Part model, mm, in its own coordinate system. Give positions to 0.01 mm unless a question says otherwise; leave off trailing zeros. Order: outer loops, then holes, each group sorted by start corner. A loop starts at its lowest first (then second) coordinate and runs counter-clockwise, first axis right, second up.
from build123d import *

# Parameters (mm, degrees)
F0_R        = 4.0800200383
F0_R_2      = 11.0109
F1_DEPTH    = 6.985
F2_T1_DEPTH = 63.627
F2_T4_ANGLE = 170.5132200492
F2_T6_ANGLE = 170.5132200492
F3_T1_DEPTH = 63.627
F3_T4_ANGLE = 170.5132200492
F3_T6_ANGLE = 170.5132200492


# Not quite as in the source:
# - a fillet or chamfer that OpenCascade refuses, or shapes differently, is made with other operations: its cross-section is extruded or revolved along the edge and cut away or added


with BuildPart() as f1:
    # F0 (on Top) → F1 (new body)
    with BuildSketch(Plane.XY):
        with BuildLine():
            Line((28.575, 15.2560200383), (-28.575, 15.2560200383))
            ThreePointArc((-28.575, 15.2560200383), (-40.9829, 0), (-28.575, -15.2560200383))
            Line((-28.575, -15.2560200383), (28.575, -15.2560200383))
            ThreePointArc((28.575, -15.2560200383), (40.9829, 0), (28.575, 15.2560200383))
        make_face()
        with Locations((-12.7, -10.16)):
            Circle(F0_R, mode=Mode.SUBTRACT)
        with Locations((12.7, -10.16)):
            Circle(F0_R, mode=Mode.SUBTRACT)
        with Locations((-25.4, 0)):
            Circle(F0_R_2, mode=Mode.SUBTRACT)
        with Locations((-12.7, 10.16)):
            Circle(F0_R, mode=Mode.SUBTRACT)
        with BuildLine():
            ThreePointArc((-11.0109, 0), (0, 11.0109), (11.0109, 0))
            ThreePointArc((11.0109, 0), (0, -11.0109), (-11.0109, 0))
        make_face(mode=Mode.SUBTRACT)
        with BuildLine():
            ThreePointArc((36.4109, 0), (25.4, -11.0109), (14.3891, 0))
            ThreePointArc((14.3891, 0), (25.4, 11.0109), (36.4109, 0))
        make_face(mode=Mode.SUBTRACT)
        with Locations((12.7, 10.16)):
            Circle(F0_R, mode=Mode.SUBTRACT)
    extrude(amount=F1_DEPTH)

    # F2: fillet of radius 0.762 on 4 edges, made by hand

    # F2_s2 → F2_t1 (cut)
    with BuildSketch(Plane.YZ.offset(-31.8135)):
        with BuildLine():
            ThreePointArc((-14.4940200383, 6.985), (-15.0328354056, 6.7618153673), (-15.2560200383, 6.223))
            Line((-15.2560200383, 6.223), (-15.2560200383, 6.985))
            Line((-15.2560200383, 6.985), (-14.4940200383, 6.985))
        make_face()
        with BuildLine():
            ThreePointArc((15.2560200383, 6.223), (15.0328354056, 6.7618153673), (14.4940200383, 6.985))
            Line((14.4940200383, 6.985), (15.2560200383, 6.985))
            Line((15.2560200383, 6.985), (15.2560200383, 6.223))
        make_face()
    extrude(amount=F2_T1_DEPTH, mode=Mode.SUBTRACT)

    # F2_s3 → F2_t4 (revolve, cut)
    with BuildSketch(Plane(origin=(-25.2263104474, -2.0932144122, 0), x_dir=(0, 0, 1), z_dir=(0.9965750492, 0.0826932365, 0))):
        with BuildLine():
            ThreePointArc((6.985, -16.921308207), (6.7618153673, -17.4601235742), (6.223, -17.683308207))
            Line((6.223, -17.683308207), (6.985, -17.683308207))
            Line((6.985, -17.683308207), (6.985, -16.921308207))
        make_face()
    revolve(axis=Axis((-25.4, 0, 6.985), (0, 0, 1)), revolution_arc=F2_T4_ANGLE, mode=Mode.SUBTRACT)

    # F2_s5 → F2_t6 (revolve, cut)
    with BuildSketch(Plane(origin=(25.2263104474, 2.0932144122, 0), x_dir=(0, 0, 1), z_dir=(-0.9965750492, -0.0826932365, 0))):
        with BuildLine():
            ThreePointArc((6.985, -16.921308207), (6.7618153673, -17.4601235742), (6.223, -17.683308207))
            Line((6.223, -17.683308207), (6.985, -17.683308207))
            Line((6.985, -17.683308207), (6.985, -16.921308207))
        make_face()
    revolve(axis=Axis((25.4, 0, 6.985), (0, 0, 1)), revolution_arc=F2_T6_ANGLE, mode=Mode.SUBTRACT)

    # F3: fillet of radius 0.762 on 4 edges, made by hand

    # F3_s2 → F3_t1 (cut)
    with BuildSketch(Plane.YZ.offset(-31.8135)):
        with BuildLine():
            ThreePointArc((15.2560200383, 0.762), (15.0328354056, 0.2231846327), (14.4940200383, 0))
            Line((14.4940200383, 0), (15.2560200383, 0))
            Line((15.2560200383, 0), (15.2560200383, 0.762))
        make_face()
        with BuildLine():
            ThreePointArc((-14.4940200383, 0), (-15.0328354056, 0.2231846327), (-15.2560200383, 0.762))
            Line((-15.2560200383, 0.762), (-15.2560200383, 0))
            Line((-15.2560200383, 0), (-14.4940200383, 0))
        make_face()
    extrude(amount=F3_T1_DEPTH, mode=Mode.SUBTRACT)

    # F3_s3 → F3_t4 (revolve, cut)
    with BuildSketch(Plane(origin=(-25.2263104474, -2.0932144122, 0), x_dir=(0, 0, 1), z_dir=(0.9965750492, 0.0826932365, 0))):
        with BuildLine():
            ThreePointArc((0, -16.921308207), (0.2231846327, -17.4601235742), (0.762, -17.683308207))
            Line((0.762, -17.683308207), (0, -17.683308207))
            Line((0, -17.683308207), (0, -16.921308207))
        make_face()
    revolve(axis=Axis((-25.4, 0, 0), (0, 0, 1)), revolution_arc=F3_T4_ANGLE, mode=Mode.SUBTRACT)

    # F3_s5 → F3_t6 (revolve, cut)
    with BuildSketch(Plane(origin=(25.2263104474, 2.0932144122, 0), x_dir=(0, 0, 1), z_dir=(-0.9965750492, -0.0826932365, 0))):
        with BuildLine():
            ThreePointArc((0, -16.921308207), (0.2231846327, -17.4601235742), (0.762, -17.683308207))
            Line((0.762, -17.683308207), (0, -17.683308207))
            Line((0, -17.683308207), (0, -16.921308207))
        make_face()
    revolve(axis=Axis((25.4, 0, 0), (0, 0, 1)), revolution_arc=F3_T6_ANGLE, mode=Mode.SUBTRACT)


solid = f1.part
Item 1: Band-saw the part on A-A on y = 0. List the corners of the cut face in (x, z) (3 decimals), plus the area to 3 significant figures.
Item 2: Drill centre lines: probe 1 along Y at (x, z) = (-12.7, 2); probe 2 along Y at (x, z) = (0, 5); probe 3 along X at (y, z) = (12, 3.25). Where is each one in solid material? Low to high.
Item 3: Pull direction X, two halves, no side cores. Call faces 1 (the face through (-9.5, 6.6, 6.985)), 2 (the face through (-40.98, 0.3, 3.45)), 3 (the face through (14.9, 3.31, 3.44)): released by +X, released by -X, zero draft, split by the parting line, or undercut.
Item 4: Band-saw the part on B-B on x = 12.5. List the corners of the cut face in (y, z) (3 decimals), plus the area to 3 significant figures.
Item 5: Drop flat-ended pins along their axis: P1, Ø7.5, axis at x = -12.7, y = -10.16, coming from the +Z side; P2, Ø4, axis at y = 7, z = 2, coming from the +X side; P3, Ø1, axis at y = 5.5, z = 2.5, coming from the -X side. Give the stop position or say it passes through.
Item 6: Band-saw the part on D-D on x = 0. List the corners of the cut face in (y, z) (3 decimals), plus the area to 3 significant figures.
Item 7: Band-saw the part on C-C on z = 5.25. List the corners of the cut face in (x, y) (3 decimals), plus the area to 3 significant figures.
Working result:
1. outline: (-40.983, 0.762) arc R0.762 ccw to (-40.221, 0) - (-36.411, 0) - (-36.411, 6.985) - (-40.221, 6.985) arc R0.762 ccw to (-40.983, 6.223) - close; (-14.389, 0) - (-11.011, 0) - (-11.011, 6.985) - (-14.389, 6.985) - close; (11.011, 0) - (14.389, 0) - (14.389, 6.985) - (11.011, 6.985) - close; (36.411, 0) - (40.221, 0) arc R0.762 ccw to (40.983, 0.762) - (40.983, 6.223) arc R0.762 ccw to (40.221, 6.985) - (36.411, 6.985) - close
1. area: 111 mm2
2. probe 1: y = -15.26 to -14.24, -6.08 to 6.08, 14.24 to 15.26
2. probe 2: y = -15.26 to -11.01, 11.01 to 15.26
2. probe 3: x = -35.34 to -16.34, -9.06 to 9.06, 16.34 to 35.34
3. face 1: zero draft
3. face 2: released by -X
3. face 3: undercut
4. outline: (-15.256, 0.762) arc R0.762 ccw to (-14.494, 0) - (-14.235, 0) - (-14.235, 6.985) - (-14.494, 6.985) arc R0.762 ccw to (-15.256, 6.223) - close; (-6.085, 0) - (6.085, 0) - (6.085, 6.985) - (-6.085, 6.985) - close; (14.235, 0) - (14.494, 0) arc R0.762 ccw to (15.256, 0.762) - (15.256, 6.223) arc R0.762 ccw to (14.494, 6.985) - (14.235, 6.985) - close
4. area: 98.8 mm2
5. P1: passes through
5. P2: stops at x = 40.16
5. P3: stops at x = -40.16
6. outline: (-15.256, 0.762) arc R0.762 ccw to (-14.494, 0) - (-11.011, 0) - (-11.011, 6.985) - (-14.494, 6.985) arc R0.762 ccw to (-15.256, 6.223) - close; (11.011, 0) - (14.494, 0) arc R0.762 ccw to (15.256, 0.762) - (15.256, 6.223) arc R0.762 ccw to (14.494, 6.985) - (11.011, 6.985) - close
6. area: 58.8 mm2
7. outline: (-28.575, -15.256) - (28.575, -15.256) arc R15.583 ccw to (28.575, 15.256) - (-28.575, 15.256) arc R15.583 ccw to start; hole circle Ø22.022 at (-25.4, 0); hole circle Ø8.16 at (-12.7, -10.16); hole circle Ø8.16 at (-12.7, 10.16); hole circle Ø22.022 at (0, 0); hole circle Ø8.16 at (12.7, -10.16); hole circle Ø8.16 at (12.7, 10.16); hole circle Ø22.022 at (25.4, 0)
7. area: 958 mm2
